Could you check a few things on this model? Use its own coordinates, in mm. A direction names the side the tool comes from. Give positions to 0.01 mm unless a question says otherwise; leave off trailing zeros. Loops run counter-clockwise (first coordinate to the right, second up) from the corner with the lowest first, then second, coordinate; pieces in that order, holes last. Notation, with made-up numbers: M 9.5,6 L 21.5,6 A35 ccw 21.5,40 Z; hole C -35.75,56.5 d9. An arc over 180 degrees is marked long. Answer in a Markdown table with one row per item. Add a question column.
1. If we section it at A-A on x = 0: List the corners of the cut face in (y, z) for me, then the cut area to 3 significant figures.
2. I'm going to push flat-ended pins straight in: pin 1 Ø1 at (x, y) = (-2.5, -9) entering from -Z; pin 2 Ø5 at (x, z) = (11, -0.5) entering from +Y; pin 3 Ø1 at (x, z) = (5, 2) entering from -Y. Where does each tip first touch, or does it pass through?
3. If we section it at D-D on x = -12: List the corners of the cut face in (y, z) for me.
4. I need wall thicknesses on line 1 along Z through (x, y) = (0, -3.25); line 2 along Z through (x, y) = (8, 12); line 3 along Y through (x, z) = (0, -2). Which ranges of each line are inside material? Lowest first, please. Write a range as from..to.
5. If we section it at B-B on y = 0: List the corners of the cut face in (x, z) for me, then the cut area to 3 significant figures.
6. If we section it at C-C on z = 1.25: List the corners of the cut face in (x, y) for me, then the cut area to 3 significant figures.
7. Thinking about a two-plate mould opening in X: for faces 1 (the cylindrical face through (-15.12, -11.59, 3.2)), 2 (the flat face through (0, 0, 0)), 3 (the flat face through (2, -1, -4.5)), 4 (the cylindrical face through (0, 2, -2)), which applies, released by +X, released by -X, zero draft, split by the parting line, or undercut?
8. Which directions (+Z, -Z, +X, -X, +Y, -Y) give clear straight access to the entire face, cutting with the end or side of a thin tool? Please do faces 5 (the cylindrical face through (-0.238, -3.191, -3.324)), 6 (the flat face through (0, 0, 6.5)), 7 (the flat face through (4, -4, 0)).
```python
from build123d import *

# Parameters (mm, degrees)
F0_R     = 19.05
F0_R_2   = 4.75
F1_DEPTH = 6.5
F2_DEPTH = 4.5
F3_R     = 2
F4_DEPTH = 4.5
F5_R     = 1.1
F6_DEPTH = 5


with BuildPart() as f1:
    # F0 (on Top) → F1 (new body)
    with BuildSketch(Plane.XY):
        Circle(F0_R)
        Circle(F0_R_2, mode=Mode.SUBTRACT)
        Circle(F0_R_2)
    extrude(amount=F1_DEPTH)

    # F0 (on Top) → F2 (join)
    with BuildSketch(Plane.XY):
        Circle(F0_R_2)
    extrude(amount=-F2_DEPTH)

    # F3 (on face) → F4 (cut)
    with BuildSketch(Plane(origin=(0, 0, -4.5), x_dir=(1, 0, 0), z_dir=(0, 0, -1))):
        Circle(F3_R)
    extrude(amount=-F4_DEPTH, mode=Mode.SUBTRACT)

    # F5 (on Front) → F6 (cut)
    with BuildSketch(Plane.XZ):
        with Locations((0, -2.25)):
            Circle(F5_R)
    extrude(amount=F6_DEPTH, mode=Mode.SUBTRACT)


solid = f1.part
```
Results:
| question | item | result |
|---|---|---|
| 1 | outline | M -19.05,0 L -4.75,0 L -4.75,-1.15 L -2,-1.15 L -2,0 L 2,0 L 2,-4.5 L 4.75,-4.5 L 4.75,0 L 19.05,0 L 19.05,6.5 L -19.05,6.5 Z; M -4.75,-4.5 L -2,-4.5 L -2,-3.35 L -4.75,-3.35 Z |
| 1 | area | 266 mm2 |
| 2 | pin 1 | z = 0 |
| 2 | pin 2 | y = 17.02 |
| 2 | pin 3 | y = -18.51 |
| 3 | outline | M -14.8,0 L 14.8,0 L 14.8,6.5 L -14.8,6.5 Z |
| 4 | line 1 | -4.5..-3.35, -1.15..6.5 |
| 4 | line 2 | 0..6.5 |
| 4 | line 3 | 2..4.75 |
| 5 | outline | M -19.05,0 L -4.75,0 L -4.75,-4.5 L -2,-4.5 L -2,0 L 2,0 L 2,-4.5 L 4.75,-4.5 L 4.75,0 L 19.05,0 L 19.05,6.5 L -19.05,6.5 Z |
| 5 | area | 272 mm2 |
| 6 | outline | C 0,0 d38.1 |
| 6 | area | 1,140 mm2 |
| 7 | face 1 | split by the parting line |
| 7 | face 2 | undercut |
| 7 | face 3 | zero draft |
| 7 | face 4 | undercut |
| 8 | face 5 | -Y |
| 8 | face 6 | +Z, +X, -X, +Y, -Y |
| 8 | face 7 | -Z |
